Verification items for the finished model (mm, model axes). A direction names the side the tool comes from. Coordinates: 2 decimals unless noted, no trailing zeros. Write each loop counter-clockwise with the first axis right and the second up, starting at its lowest first coordinate (ties: lowest second). Pieces come first, ordered by that corner, then holes. Notation, with made-up numbers: (-38, 57) -> (16, 57) arc R18 cw to (16, 78) -> close; hole circle Ø6 at (-30, 22.25). An arc over 180 degrees is marked (long way). Write item = value, one per line. Start each with the question number.
(1) Section check B-B (x = -32). Record the cut outline in (y, z).
(2) Section check C-C (y = -18). Record the cut outline in (x, z), plus the area to 3 significant figures.
(3) Material ranges on probe 1 along Y at (x, z) = (8, -43.5); probe 2 along X at (y, z) = (13.5, -14.5); probe 3 along Z at (x, y) = (42, 34), recorded low to high. Write a range as [from, to].
(4) Set-up check for faces 1 (the face through (-1, 1, -69.85)), 2 (the face through (-6, -39, 0)): record each of +Z, -Z, +X, -X, +Y, -Y from which the full face is reachable in a straight line by a thin tool's end or side.
(5) Section check A-A (z = -24.5). Record the cut outline in (x, y).
(6) Mould release check, pull along X, two halves, no side actions. Record for faces 3 (the face through (76.2, -1, -38)), 4 (the face through (-1, -44.45, -38)), 5 (the face through (1, 38.1, -34)), 6 (the face through (-1, -38.1, -34)): released by +X, released by -X, zero draft, split by the parting line, or undercut.
```python
from build123d import *

# Parameters (mm, degrees)
F1_DEPTH = 76.2
F2_DEPTH = 69.85


with BuildPart() as f1:
    # F0 (on Top) → F1 (new body)
    with BuildSketch(Plane.XY):
        Polygon((-69.85, -38.1), (0, -38.1), (69.85, -38.1), (69.85, 38.1), (0, 38.1), (-69.85, 38.1), align=None)
        Polygon((-76.2, -44.45), (0, -44.45), (0, -38.1), (-69.85, -38.1), (-69.85, 38.1), (0, 38.1), (0, 44.45), (-76.2, 44.45), align=None)
        Polygon((0, -44.45), (76.2, -44.45), (76.2, 44.45), (0, 44.45), (0, 38.1), (69.85, 38.1), (69.85, -38.1), (0, -38.1), align=None)
    extrude(amount=-F1_DEPTH)

    # F0 (on Top) → F2 (cut)
    with BuildSketch(Plane.XY):
        Polygon((-69.85, -38.1), (0, -38.1), (69.85, -38.1), (69.85, 38.1), (0, 38.1), (-69.85, 38.1), align=None)
    extrude(amount=-F2_DEPTH, mode=Mode.SUBTRACT)


solid = f1.part
```
Response:
q1.outline = (-44.45, -76.2) -> (44.45, -76.2) -> (44.45, 0) -> (38.1, 0) -> (38.1, -69.85) -> (-38.1, -69.85) -> (-38.1, 0) -> (-44.45, 0) -> close
q2.outline = (-76.2, -76.2) -> (76.2, -76.2) -> (76.2, 0) -> (69.85, 0) -> (69.85, -69.85) -> (-69.85, -69.85) -> (-69.85, 0) -> (-76.2, 0) -> close
q2.area = 1,850 mm2
q3.probe_1 = [-44.45, -38.1], [38.1, 44.45]
q3.probe_2 = [-76.2, -69.85], [69.85, 76.2]
q3.probe_3 = [-76.2, -69.85]
q4.face_1 = +Z
q4.face_2 = +Z, +X, -X, +Y, -Y
q5.outline = (-76.2, -44.45) -> (76.2, -44.45) -> (76.2, 44.45) -> (-76.2, 44.45) -> close; hole (-69.85, -38.1) -> (69.85, -38.1) -> (69.85, 38.1) -> (-69.85, 38.1) -> close
q6.face_3 = released by +X
q6.face_4 = zero draft
q6.face_5 = undercut
q6.face_6 = undercut
